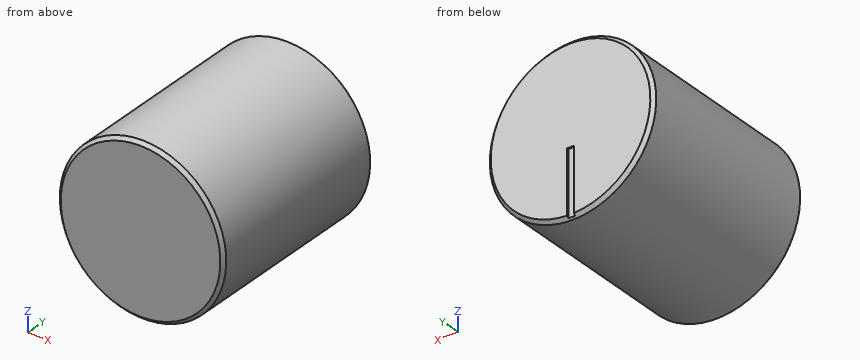
```python
from build123d import *

# Parameters (mm, degrees)
SKETCH1_R           = 6.25
BOSS_EXTRUDE1_DEPTH = 15
CHAMFER1_SIZE       = 0.254
SKETCH2_W           = 0.508
SKETCH2_H           = 4.943764677
CUT_EXTRUDE1_DEPTH  = 0.127


with BuildPart() as part:
    # Sketch1 → Boss-Extrude1 (new body)
    with BuildSketch(Plane(origin=(0, 0, 0), x_dir=(1, 0, 0), z_dir=(0, 1, 0))):
        with Locations(Location((0, 0, 0), (0, 0, 270))):
            Circle(SKETCH1_R)
    extrude(amount=BOSS_EXTRUDE1_DEPTH)

    # Chamfer1
    chamfer1_edges = [part.edges().sort_by_distance(p)[0] for p in [
        (0, 0, -6.25),
        (0, 15, -6.25),
    ]]
    chamfer(chamfer1_edges, length=CHAMFER1_SIZE)

    # Sketch2 → Cut-Extrude1 (cut)
    with BuildSketch(Plane(origin=(0, 15, 0), x_dir=(1, 0, 0), z_dir=(0, 1, 0))):
        with Locations((0, 3.741882338)):
            Rectangle(SKETCH2_W, SKETCH2_H)
    extrude(amount=-CUT_EXTRUDE1_DEPTH, mode=Mode.SUBTRACT)


solid = part.part
```
Here's how the part is built. I have some questions about the finished solid (model axes, mm). Round coordinates to 2 decimals unless told otherwise and drop trailing zeros. Order: outer loops, then holes, each group sorted by start corner. A loop starts at its lowest first (then second) coordinate and runs counter-clockwise, first axis right, second up. Notation, with made-up numbers: (26.25, 1) -> (38.25, 1) arc R19 ccw to (38.25, 8) -> close; hole circle Ø2 at (66.5, 52). An arc over 180 degrees is marked (long way). Use a Markdown table: item, result. Add a question column.
(1) Suppose I cut it at A-A, the plane y = 5.5. Please give me the cut outline in (x, z).
(2) I need wall thicknesses on line 1 along X through (y, z) = (11.5, -5.25); line 2 along X through (y, z) = (4.25, -1); line 3 along Z through (x, y) = (5.5, 13.75). Which ranges of each line are inside material? Lowest first, please.
(3) For pin 1 Ø1 at (y, z) = (13.5, 3.5) entering from +X; pin 2 Ø1.5 at (x, y) = (-3, 2) entering from +Z; pin 3 Ø6 at (y, z) = (7.5, 4.5) entering from -X, each with a flat end and sliding along its axis, tell me the tip position at first contact or that it passes through.
Verdict:
| question | item | result |
|---|---|---|
| 1 | outline | circle Ø12.5 at (0, 0) |
| 2 | line 1 | -3.39 to 3.39 |
| 2 | line 2 | -6.17 to 6.17 |
| 2 | line 3 | -2.97 to 2.97 |
| 3 | pin 1 | x = 5.48 |
| 3 | pin 2 | z = 5.83 |
| 3 | pin 3 | x = -6.07 |
